```python
from build123d import *

# Parameters (mm, degrees)
SKETCH2_R           = 15
BOSS_EXTRUDE1_DEPTH = 16


with BuildPart() as part:
    # Sketch2 → Boss-Extrude1 (new body)
    with BuildSketch(Plane.XY):
        Polygon((18.953313646, 37.5), (50, 0.5), (50, -19.5), (20, -19.5), (20, -29.5), (50, -29.5), (50, -37.5), (-13, -37.5), (-13, -32.5), (-38, -32.5), (-38, -37.5), (-50, -37.5), (-50, -27.5), (-40, -27.5), (-40, -7.5), (-30, -7.5), (-30, 17.5), (-14, 17.5), (-14, 37.5), align=None)
        with Locations((10, 7.5)):
            Circle(SKETCH2_R, mode=Mode.SUBTRACT)
    extrude(amount=BOSS_EXTRUDE1_DEPTH)


solid = part.part
```
The listing builds one solid part. Answer for the finished solid, in the listing's coordinates (mm). A direction names the side the tool comes from. Coordinates: 2 decimals unless noted, no trailing zeros. Order: outer loops, then holes, each group sorted by start corner. A loop starts at its lowest first (then second) coordinate and runs counter-clockwise, first axis right, second up. Notation, with made-up numbers: M -17,13.5 L -11,13.5 A7 ccw -11,18.5 Z; hole C 81,46 d10. An arc over 180 degrees is marked long. Answer as a JSON object with one key per item and string values. Group by question number.
1. Section C-C on z = 13.25 is taken. Write down the section's boundary in (x, y).
2. Flat-ended cylindrical pins translate along their axes: P1, Ø1, axis at y = 28.5, z = 4, coming from the -X side; P2, Ø5, axis at x = -35, z = 4.5, coming from the +Y side; P3, Ø5, axis at x = -21.5, z = 6.5, coming from the +Y side. Find the tip coordinate at first contact, or state that the pin passes through.
3. Section A-A on x = 10 is taken. Write down the section's boundary in (y, z), then the cut area to 3 significant figures.
4. Section D-D on y = -10.5 is taken. Write down the section's boundary in (x, z).
5. Determine the mould class of faces 1 (the flat face through (-22, 17.5, 8)), 2 (the flat face through (35, -19.5, 8)), 3 (the flat face through (-25, -32.5, 8)), 4 (the flat face through (-40, -18, 8)) for opening direction Y: released by +Y, released by -Y, zero draft, split by the parting line, or undercut.
6. Section B-B on y = 7.5 is taken. Write down the section's boundary in (x, z).
7. Straight lines are drawn through the part: line 1 (Y direction, x = 10, z = 5); line 2 (Y direction, x = -39.5, z = 14.75); line 3 (X direction, y = 3.5, z = 5.75). For each, find the intervals that lie inside material, in ascending order.
8. A tool of negligible diameter and unlimited length cuts with its end or side. For faces 5 (the flat face through (19, -37.5, 8)), 6 (the flat face through (-38, -35, 8)), 7 (the flat face through (35, -29.5, 8)), 8 (the flat face through (-30, 5, 8)), from which of +Z, -Z, +X, -X, +Y, -Y can it reach the whole face along a straight path? Write none if from no direction.
Values follow:
{
 "1": {"outline": "M -50,-37.5 L -38,-37.5 L -38,-32.5 L -13,-32.5 L -13,-37.5 L 50,-37.5 L 50,-29.5 L 20,-29.5 L 20,-19.5 L 50,-19.5 L 50,0.5 L 18.95,37.5 L -14,37.5 L -14,17.5 L -30,17.5 L -30,-7.5 L -40,-7.5 L -40,-27.5 L -50,-27.5 Z; hole C 10,7.5 d30"},
 "2": {"P1": "x = -14", "P2": "y = -7.5", "P3": "y = 17.5"},
 "3": {"outline": "M -37.5,0 L -7.5,0 L -7.5,16 L -37.5,16 Z; M 22.5,0 L 37.5,0 L 37.5,16 L 22.5,16 Z", "area": "720 mm2"},
 "4": {"outline": "M -40,0 L 50,0 L 50,16 L -40,16 Z"},
 "5": {"face 1": "released by +Y", "face 2": "undercut", "face 3": "released by -Y", "face 4": "zero draft"},
 "6": {"outline": "M -30,0 L -5,0 L -5,16 L -30,16 Z; M 25,0 L 44.13,0 L 44.13,16 L 25,16 Z"},
 "7": {"line 1": "-37.5 to -7.5, 22.5 to 37.5", "line 2": "-37.5 to -7.5", "line 3": "-30 to -4.46, 24.46 to 47.48"},
 "8": {"face 5": "+Z, -Z, +X, -X, -Y", "face 6": "+Z, -Z, -Y", "face 7": "+Z, -Z, +X", "face 8": "+Z, -Z, -X, +Y"}
}
